Model file for the job. Use its own axes, mm. Round coordinates to 2 decimals unless told otherwise and drop trailing zeros. Order: outer loops, then holes, each group sorted by start corner. A loop starts at its lowest first (then second) coordinate and runs counter-clockwise, first axis right, second up. Notation, with made-up numbers: (-12.5, 87) -> (46.5, 87) arc R18 cw to (46.5, 121) -> close; hole circle Ø6 at (89.25, 63). An arc over 180 degrees is marked (long way). Put each result on its own line as item: value. Start each with the question number.
Q1. Cut at A-A, the plane z = -413. List the corners of the cut face in (x, y), and give its area (3 significant figures).
Q2. Cut at B-B, the plane x = 396.5. List the corners of the cut face in (y, z), and give its area (3 significant figures).
Q3. Probe L1, parallel to Y at x = 580, z = -7; L2, parallel to X at y = 41.5, z = -445.5; L3, parallel to Z at x = 462, y = 46.5. List the from-to ranges inside material, lowest first.
from build123d import *

# Parameters (mm, degrees)
SKETCH2_W           = 1626.4
SKETCH2_H           = 914.4
BOSS_EXTRUDE1_DEPTH = 100
SHELL1_T            = -10
SKETCH3_W           = 1526.4
SKETCH3_H           = 814.4
CUT_EXTRUDE1_DEPTH  = 1868.994732327
SKETCH5_R           = 4
CUT_EXTRUDE2_DEPTH  = 1869.503229861
SKETCH6_R           = 4
CUT_EXTRUDE3_DEPTH  = 1869.503229861
SKETCH7_R           = 4
CUT_EXTRUDE4_DEPTH  = 1869.503229861


with BuildPart() as part:
    # Sketch2 → Boss-Extrude1 (new body)
    with BuildSketch(Plane(origin=(0, 0, 0), x_dir=(1, 0, 0), z_dir=(0, 1, 0))):
        with Locations((813.2, 457.2)):
            Rectangle(SKETCH2_W, SKETCH2_H)
    extrude(amount=BOSS_EXTRUDE1_DEPTH)

    # Shell1
    shell1_openings = [part.faces().sort_by_distance(p)[0] for p in [
        (813.2, 100, -457.2),
    ]]
    offset(amount=SHELL1_T, openings=shell1_openings, kind=Kind.INTERSECTION)

    # Sketch3 → Cut-Extrude1 (cut, through all)
    with BuildSketch(Plane(origin=(0, 10, 0), x_dir=(1, 0, 0), z_dir=(0, 1, 0))):
        with Locations((813.2, 457.2)):
            Rectangle(SKETCH3_W, SKETCH3_H)
    extrude(amount=-CUT_EXTRUDE1_DEPTH, mode=Mode.SUBTRACT)

    # Sketch5 → Cut-Extrude2 (cut, through all)
    with BuildSketch(Plane(origin=(1626.4, 0, 0), x_dir=(0, 0, -1), z_dir=(1, 0, 0))):
        with Locations((7.85, 50)):
            Circle(SKETCH5_R)
    extrude(amount=-CUT_EXTRUDE2_DEPTH, mode=Mode.SUBTRACT)

    # Sketch6 → Cut-Extrude3 (cut, through all)
    with BuildSketch(Plane(origin=(1626.4, 0, 0), x_dir=(0, 0, -1), z_dir=(1, 0, 0))):
        with Locations((7.85, 66.28)):
            Circle(SKETCH6_R)
    extrude(amount=-CUT_EXTRUDE3_DEPTH, mode=Mode.SUBTRACT)

    # Sketch7 → Cut-Extrude4 (cut, through all)
    with BuildSketch(Plane(origin=(1626.4, 0, 0), x_dir=(0, 0, -1), z_dir=(1, 0, 0))):
        with Locations((7.85, 33.72)):
            Circle(SKETCH7_R)
    extrude(amount=-CUT_EXTRUDE4_DEPTH, mode=Mode.SUBTRACT)


solid = part.part
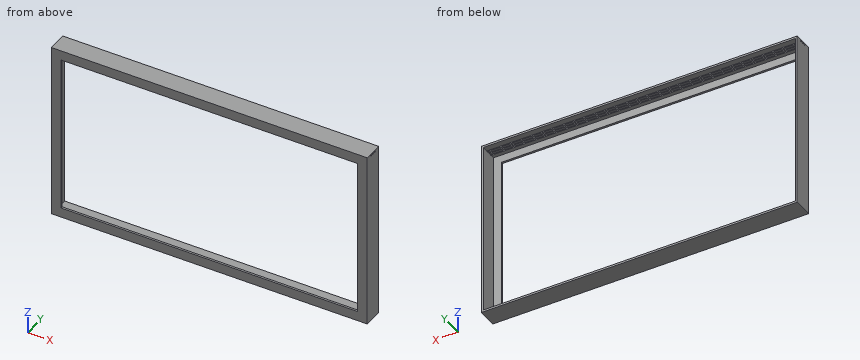
Ans:
1. outline: (0, 0) -> (50, 0) -> (50, 10) -> (10, 10) -> (10, 100) -> (0, 100) -> close; (1576.4, 0) -> (1626.4, 0) -> (1626.4, 100) -> (1616.4, 100) -> (1616.4, 10) -> (1576.4, 10) -> close
1. area: 2,800 mm^2
2. outline: (0, -914.4) -> (100, -914.4) -> (100, -904.4) -> (10, -904.4) -> (10, -864.4) -> (0, -864.4) -> close; (0, -50) -> (10, -50) -> (10, -10) -> (30.35, -10) arc R4 cw (long way) to (37.09, -10) -> (46.63, -10) arc R4 cw (long way) to (53.37, -10) -> (62.91, -10) arc R4 cw (long way) to (69.65, -10) -> (100, -10) -> (100, 0) -> (0, 0) -> close
2. area: 2,680 mm^2
3. L1: y = 0 to 29.81, 37.63 to 46.09, 53.91 to 62.37, 70.19 to 100
3. L2: x = 0 to 10, 1616.4 to 1626.4
3. L3: z = -914.4 to -904.4, -10 to -9.79, -5.91 to 0
